Work out the finished part from the listing and answer in its coordinate system (mm). Face numbers are marked on the shaded views. Round coordinates to 2 decimals unless told otherwise and drop trailing zeros. Order: outer loops, then holes, each group sorted by start corner. A loop starts at its lowest first (then second) coordinate and runs counter-clockwise, first axis right, second up. Notation, with made-up numbers: M 45.25,23 L 53.25,23 A11 ccw 53.25,27 Z; hole C 48,11 d10. An arc over 180 degrees is marked long. Answer as a JSON object with one key per item and string values. Group by question number.
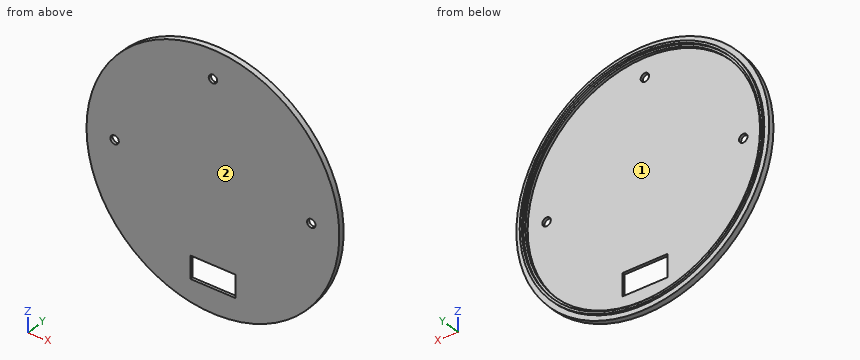
Autodesk Inventor part; units mm, degrees
ref_plane "YZ Plane" through (0, 0, 0) normal (1, 0, 0) x (0, 1, 0)
ref_plane "XZ Plane" through (0, 0, 0) normal (0, 1, 0) x (-1, 0, 0)
ref_plane "XY Plane" through (0, 0, 0) normal (0, 0, 1) x (1, 0, 0)
sketch "Sketch1" plane through (0, 0, 0) normal (0, 1, 0) x (-1, 0, 0)
  circle A0 centre (0, 0) radius 45
  dimension "d0" = 90
extrude "Extrusion1" add sketch "Sketch1" along normal blind 2
sketch "Sketch2" plane through (0, 2, 0) normal (0, 1, 0) x (1, 0, 0)
  circle A0 centre (0, 0) radius 45
  circle A1 centre (0, 0) radius 42.5
  circle A2 centre (0, 0) radius 41.75
  circle A3 centre (0, 0) radius 43.25
  dimension "d3" = 2.5
  dimension "d4" = 0.75
  dimension "d5" = 0.75
extrude "Extrusion2" cut sketch "Sketch2" against normal blind 1 contours A2
extrude "Extrusion3" add sketch "Sketch2" along normal blind 0.75 contours A3
sketch "Sketch3" plane through (0, 1, 0) normal (0, 1, 0) x (1, 0, 0)
  circle A0 centre (0, 0) radius 40 construction
  line L0 (8, 36.45) -> (-8, 36.45)
  line L1 (-8, 36.45) -> (-8, 28.45)
  line L2 (-8, 28.45) -> (8, 28.45)
  line L3 (8, 28.45) -> (8, 36.45)
  circle A1 centre (35, 0) radius 1.5
  circle A2 centre (0, -35) radius 1.5
  circle A3 centre (-35, 0) radius 1.5
  line L4 (40, 0) -> (-40, 0) construction
  line L5 (0, 0) -> (0, -40) construction
  line L6 (0, 0) -> (0, 40) construction
  point P0 (0, 36.45)
  dimension "d10" = 80
  dimension "d11" = 5
  dimension "d12" = 3
  dimension "d13" = 3
  dimension "d14" = 5
  dimension "d15" = 3
  dimension "d16" = 5
  dimension "d17" = 16
  dimension "d18" = 8
  dimension "d21" = 36.45
extrude "Extrusion5" cut sketch "Sketch3" against normal through all contours L3 L2 L1 L0
extrude "Extrusion6" cut sketch "Sketch3" against normal through all contours A1 | A2 | A3
properties part number "ROUNDTOPCOVER"
Item 1: Each of these flat-tipped pins is pushed along its axis until it touches: pin 1 (0.5 mm diameter, centred on y = 0.5, z = -31, fed in from -X); pin 2 (0.8 mm diameter, centred on x = 1.5, y = 0.5, fed in from +Z); pin 3 (0.8 mm diameter, centred on x = 0.5, y = 0.5, fed in from -Z); pin 4 (2.5 mm diameter, centred on x = 0, z = 35, fed in from -Y). Where does it stop, or does it pass through?
Item 2: Consider L1, parallel to Z at x = 0, y = 0.8; L2, parallel to X at y = 2.6, z = 0; L3, parallel to Z at x = 0, y = 1.7. Determine where each line is inside the solid, lowest interval first.
Item 3: Find section B-B (y = 0.5). Give the vertices of the cut face in (x, z), and give its area (3 significant figures).
Item 4: Find section C-C (x = 0). Give the vertices of the cut face in (y, z), and give its area (3 significant figures).
Item 5: The mould has two halves that part along Z. Classify the marked faces 1 and 2: +Z half, -Z half, draft (parallel to the pull), parting line (faces both ways), or undercut.
Item 6: Find section D-D (x = 35). Give the vertices of the cut face in (y, z).
Item 7: Find section A-A (z = 0). Give the vertices of the cut face in (x, y), and give its area (3 significant figures).
Responses:
{
 "1": {"pin 1": "stops at x = -32.85", "pin 2": "stops at z = 44.99", "pin 3": "stops at z = -45", "pin 4": "passes through"},
 "2": {"L1": "z = -45 to -36.45, -28.45 to 33.5, 36.5 to 45", "L2": "x = -43.25 to -42.5, 42.5 to 43.25", "L3": "z = -45 to -41.75, 41.75 to 45"},
 "3": {"outline": "C 0,0 d90; hole C -35,0 d3; hole M -8,-36.45 L 8,-36.45 L 8,-28.45 L -8,-28.45 Z; hole C 0,35 d3; hole C 35,0 d3", "area": "6,210 mm^2"},
 "4": {"outline": "M 0,-45 L 2,-45 L 2,-43.25 L 2.75,-43.25 L 2.75,-42.5 L 2,-42.5 L 2,-41.75 L 1,-41.75 L 1,-36.45 L 0,-36.45 Z; M 0,-28.45 L 1,-28.45 L 1,33.5 L 0,33.5 Z; M 0,36.5 L 1,36.5 L 1,41.75 L 2,41.75 L 2,42.5 L 2.75,42.5 L 2.75,43.25 L 2,43.25 L 2,45 L 0,45 Z", "area": "86.6 mm^2"},
 "5": {"face 1": "undercut", "face 2": "draft"},
 "6": {"outline": "M 0,-28.28 L 2,-28.28 L 2,-25.41 L 2.75,-25.41 L 2.75,-24.11 L 2,-24.11 L 2,-22.76 L 1,-22.76 L 1,-1.5 L 0,-1.5 Z; M 0,1.5 L 1,1.5 L 1,22.76 L 2,22.76 L 2,24.11 L 2.75,24.11 L 2.75,25.41 L 2,25.41 L 2,28.28 L 0,28.28 Z"},
 "7": {"outline": "M -45,0 L -36.5,0 L -36.5,1 L -41.75,1 L -41.75,2 L -42.5,2 L -42.5,2.75 L -43.25,2.75 L -43.25,2 L -45,2 Z; M -33.5,0 L 33.5,0 L 33.5,1 L -33.5,1 Z; M 36.5,0 L 45,0 L 45,2 L 43.25,2 L 43.25,2.75 L 42.5,2.75 L 42.5,2 L 41.75,2 L 41.75,1 L 36.5,1 Z", "area": "91.6 mm^2"}
}
